Could you check a few things on this model? Use its own coordinates, in mm. Face numbers are marked on the shaded views. A direction names the side the tool comes from. Give positions to 0.01 mm unless a question says otherwise; leave off trailing zeros. Order: outer loops, then holes, each group sorted by start corner. A loop starts at its lowest first (then second) coordinate and runs counter-clockwise, first axis right, second up. Notation, with made-up numbers: (85, -6.5) -> (101, -6.5) arc R19 cw to (101, -2.5) -> close; hole circle Ø5 at (68, 9.5). An arc over 180 degrees is marked (long way). Write each question's results on one line, items separated by ' | '.
```python
from build123d import *

# Parameters (mm, degrees)
F0_W     = 13
F0_H     = 27
F0_R     = 3
F1_DEPTH = 20
F3_DEPTH = 13.5
F4_R     = 10


with BuildPart() as f1:
    # F0 (on Front) → F1 (new body)
    with BuildSketch(Plane.XZ):
        with Locations((-30, 0)):
            Rectangle(F0_W, F0_H)
        with Locations((-30, -8)):
            Circle(F0_R, mode=Mode.SUBTRACT)
        with Locations((-30, 8)):
            Circle(F0_R, mode=Mode.SUBTRACT)
        with Locations((30, 0)):
            Rectangle(F0_W, F0_H)
        with Locations((30, -8)):
            Circle(F0_R, mode=Mode.SUBTRACT)
        with Locations((30, 8)):
            Circle(F0_R, mode=Mode.SUBTRACT)
    extrude(amount=F1_DEPTH)

    # F2 (on Top) → F3 (join, symmetric)
    with BuildSketch(Plane.XY):
        Polygon((36.5, -20), (-36.5, -20), (-17.594396, -47), (17.594396, -47), align=None)
    extrude(amount=F3_DEPTH, both=True)

    # F4
    f4_edges = [f1.edges().sort_by_distance(p)[0] for p in [
        (-23.5, -20, 0),
        (23.5, -20, 0),
        (-17.594396, -47, 0),
        (17.594396, -47, 0),
        (-36.5, -20, 0),
        (36.5, -20, 0),
    ]]
    fillet(f4_edges, radius=F4_R)


solid = f1.part
```
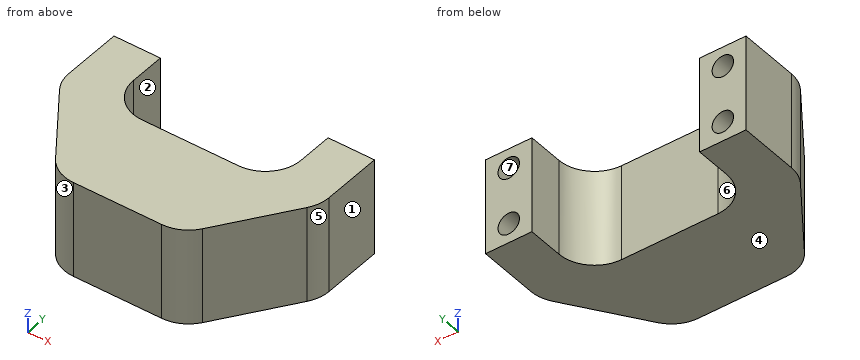
Q1. Suppose I cut it at D-D on x = 30. Please give me the cut outline in (y, z), and give its area (3 significant figures).
Here are the results:
outline: (-29.28, -13.5) -> (0, -13.5) -> (0, -11) -> (-20, -11) -> (-20, -5) -> (0, -5) -> (0, 5) -> (-20, 5) -> (-20, 11) -> (0, 11) -> (0, 13.5) -> (-29.28, 13.5) -> close | area: 551 mm²
Q2. I need wall thicknesses on line 1 along Z through (x, y) = (30, -9.5); line 2 along X through (y, z) = (-2, 1.75); line 3 along X through (y, z) = (-17, 6). Which ranges of each line are inside material? Lowest first, please.
Here are the results:
line 1: z = -13.5 to -11, -5 to 5, 11 to 13.5 | line 2: x = -36.5 to -23.5, 23.5 to 36.5 | line 3: x = -36.5 to -32.24, -27.76 to -20.64, 20.64 to 27.76, 32.24 to 36.5
Q3. For the marked faces 5, 6 and 7, which set-ups out of +Z, -Z, +X, -X, +Y, -Y let a thin tool reach every point of the face, with its end or its side?
Here are the results:
face 5: +Z, -Z, +X, -Y | face 6: +Z, -Z, +Y | face 7: +Y
Q4. I'm going to push flat-ended pins straight in: pin 1 Ø7 at (x, z) = (30, 8) entering from -Y; pin 2 Ø12 at (x, z) = (-8, -2) entering from +Y; pin 3 Ø5 at (x, z) = (-30, -8) entering from -Y. Where does each tip first touch, or does it pass through?
Here are the results:
pin 1: stops at y = -34.28 | pin 2: stops at y = -19.99 | pin 3: stops at y = -32.85
Q5. Suppose I cut it at C-C on y = -33.5. Please give me the cut outline in (x, z), and give its area (3 significant figures).
Here are the results:
outline: (-27.05, -13.5) -> (27.05, -13.5) -> (27.05, 13.5) -> (-27.05, 13.5) -> close | area: 1,460 mm²
Q6. Suppose I cut it at A-A on z = -8. Please give me the cut outline in (x, y), and give its area (3 significant figures).
Here are the results:
outline: (-36.5, -16.85) arc R10 ccw to (-34.69, -22.58) -> (-20.58, -42.74) arc R10 ccw to (-12.39, -47) -> (12.39, -47) arc R10 ccw to (20.58, -42.74) -> (34.69, -22.58) arc R10 ccw to (36.5, -16.85) -> (36.5, 0) -> (33, 0) -> (33, -20) -> (27, -20) -> (27, 0) -> (23.5, 0) -> (23.5, -10) arc R10 cw to (13.5, -20) -> (-13.5, -20) arc R10 cw to (-23.5, -10) -> (-23.5, 0) -> (-27, 0) -> (-27, -20) -> (-33, -20) -> (-33, 0) -> (-36.5, 0) -> close | area: 1,770 mm²
Q7. Suppose I cut it at B-B on x = 11. Please give me the cut outline in (y, z).
Here are the results:
outline: (-47, -13.5) -> (-20, -13.5) -> (-20, 13.5) -> (-47, 13.5) -> close
Q8. Thinking about a two-plate mould opening in X: for the marked faces 1, 2, 3 and 4, which applies, +X half, -X half, draft (parallel to the pull), parting line (faces both ways), or undercut?
Here are the results:
face 1: +X half | face 2: undercut | face 3: -X half | face 4: draft
